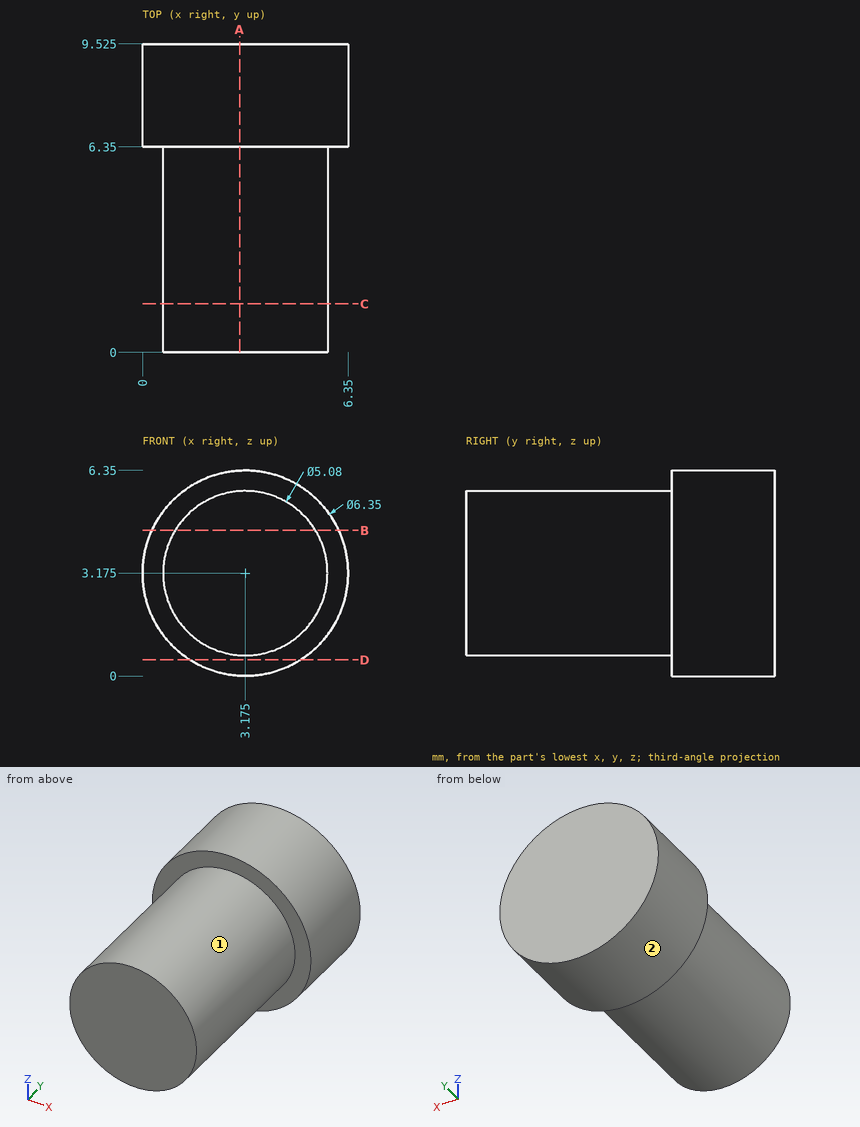
Here's the drawing with two shaded views (mm, measured from the low corner). I have some questions. A direction names the side the tool comes from. Round coordinates to 2 decimals unless told otherwise and drop trailing zeros. Write each loop counter-clockwise with the first axis right and the second up, starting at its lowest first coordinate (ties: lowest second). Pieces come first, ordered by that corner, then holes.
(1) For pin 1 (1.5 mm diameter, centred on y = 6, z = 5, fed in from +X); pin 2 (1.5 mm diameter, centred on x = 1.5, y = 3, fed in from -Z); pin 3 (1 mm diameter, centred on x = 3.5, y = 3.5, fed in from -Z) (3 decimals), each with a flat end and sliding along its axis, tell me the tip position at first contact or that it passes through.
Findings below:
pin 1: stops at x = 6.13
pin 2: stops at z = 0.81
pin 3: stops at z = 0.635
(2) Suppose I cut it at D-D on z = 0.5. Write out the boundary of the cut face in (x, y) (3 decimals), and give its area (3 significant figures).
Findings below:
outline: (1.465, 6.35) - (4.885, 6.35) - (4.885, 9.525) - (1.465, 9.525) - close
area: 10.9 mm2
(3) If I drill on probe 1 along Y at (x, z) = (2, 6) (3 decimals); probe 2 along Z at (x, y) = (4.25, 9); probe 3 along Z at (x, y) = (2.75, 8.25), over which ranges is the centre line in solid material (lowest first)?
Findings below:
probe 1: y = 6.35 to 9.525
probe 2: z = 0.19 to 6.16
probe 3: z = 0.03 to 6.32
(4) Suppose I cut it at C-C on y = 1.5. Write out the boundary of the cut face in (x, z) (3 decimals).
Findings below:
outline: circle Ø5.08 at (3.175, 3.175)
(5) Suppose I cut it at B-B on z = 4.5. Write out the boundary of the cut face in (x, y) (3 decimals), and give its area (3 significant figures).
Findings below:
outline: (0.29, 6.35) - (1.008, 6.35) - (1.008, 0) - (5.342, 0) - (5.342, 6.35) - (6.06, 6.35) - (6.06, 9.525) - (0.29, 9.525) - close
area: 45.8 mm2
(6) Which directions (+Z, -Z, +X, -X, +Y, -Y) give clear straight access to the entire face, cutting with the end or side of a thin tool? Please do the marked faces 1 and 2.
Findings below:
face 1: -Y
face 2: +Y, -Y
(7) Suppose I cut it at A-A on x = 3. Write out the boundary of the cut face in (y, z) (3 decimals).
Findings below:
outline: (0, 0.641) - (6.35, 0.641) - (6.35, 0.005) - (9.525, 0.005) - (9.525, 6.345) - (6.35, 6.345) - (6.35, 5.709) - (0, 5.709) - close
